Part print with two shaded views. Sizes in mm from the minimum x, y, z corner. A direction names the side the tool comes from. Coordinates: 2 decimals unless noted, no trailing zeros. Order: outer loops, then holes, each group sorted by start corner. A loop starts at its lowest first (then second) coordinate and runs counter-clockwise, first axis right, second up. Notation, with made-up numbers: (25.25, 54) - (37.25, 54) arc R28 ccw to (37.25, 90) - close; hole circle Ø4 at (67.25, -31). An arc over 180 degrees is marked (long way). Return JSON: item names as keys, results as strings.
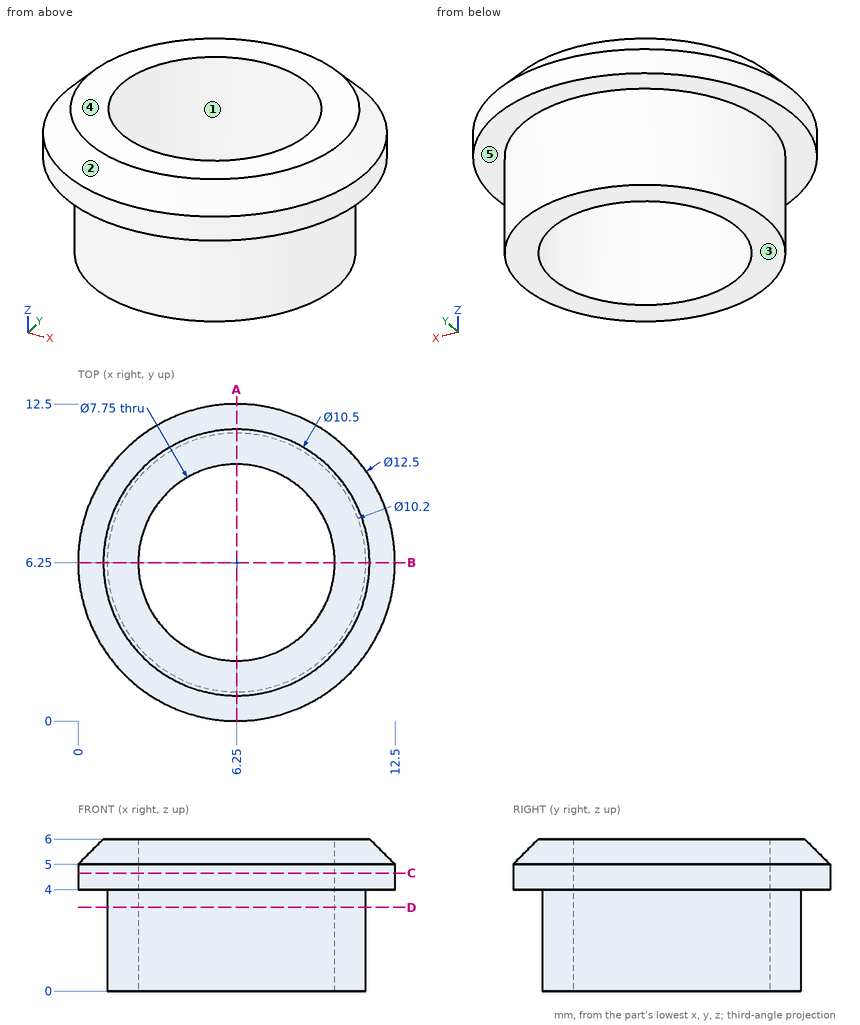
Item 1: Band-saw the part on C-C, the plane z = 4.65. List the corners of the cut face in (x, y) (3 decimals), then the cut area to 3 significant figures.
Findings below:
{"outline": "circle Ø12.5 at (6.25, 6.25); hole circle Ø7.75 at (6.25, 6.25)", "area": "75.5 mm²"}
Item 2: Band-saw the part on A-A, the plane x = 6.25. List the corners of the cut face in (y, z) (3 decimals).
Findings below:
{"outline": "(0, 4) - (1.15, 4) - (1.15, 0) - (2.375, 0) - (2.375, 6) - (1, 6) - (0, 5) - close; (10.125, 0) - (11.35, 0) - (11.35, 4) - (12.5, 4) - (12.5, 5) - (11.5, 6) - (10.125, 6) - close"}
Item 3: Mould opens along X. For the marked faces 1, 2 and 3 say: released by +X, released by -X, zero draft, split by the parting line, or undercut.
Findings below:
{"face 1": "undercut", "face 2": "split by the parting line", "face 3": "zero draft"}
Item 4: Drop flat-ended pins along their axis: P1, Ø1.5, axis at x = 2, y = 1.5, coming from the -Z side; P2, Ø1, axis at x = 4, z = 2, coming from the -Y side. Give the stop position or say it passes through.
Findings below:
{"P1": "stops at z = 4", "P2": "stops at y = 1.46"}
Item 5: Which spindle directions (+Z, -Z, +X, -X, +Y, -Y) get a long thin tool onto all of the face, cutting with end or side? Do the marked faces 4 and 5. Say none if no direction does.
Findings below:
{"face 4": "+Z, +X, -X, +Y, -Y", "face 5": "-Z"}
Item 6: Wall check: L1, parallel to Y at x = 6.25, z = 3.85 (3 decimals); L2, parallel to Y at x = 6.25, z = 4.25 (3 decimals); L3, parallel to X at y = 6, z = 5.1. Give the ranges that are in metal, low to high. Write a range as [from, to].
Findings below:
{"L1": "y = [1.15, 2.375], [10.125, 11.35]", "L2": "y = [0, 2.375], [10.125, 12.5]", "L3": "x = [0.11, 2.38], [10.12, 12.39]"}
Item 7: Band-saw the part on D-D, the plane z = 3.3. List the corners of the cut face in (x, y) (3 decimals).
Findings below:
{"outline": "circle Ø10.2 at (6.25, 6.25); hole circle Ø7.75 at (6.25, 6.25)"}
